from build123d import *

# Parameters (mm, degrees)
F0_R     = 11.125
F1_DEPTH = 7.5
F2_SIZE  = 1.524


with BuildPart() as f1:
    # F0 (on Top) → F1 (new body)
    with BuildSketch(Plane.XY):
        with BuildLine():
            ThreePointArc((13.1013648304, -5.7309894069), (13.9971339401, -2.9274974745), (14.3, 0))
            ThreePointArc((14.3, 0), (10.6581248351, 9.5338541524), (1.5875, 14.2116094708))
            Line((1.5875, 14.2116094708), (1.5875, 12.7125))
            Line((1.5875, 12.7125), (-1.5875, 12.7125))
            Line((-1.5875, 12.7125), (-1.5875, 14.2116094708))
            ThreePointArc((-1.5875, 14.2116094708), (-12.3841632741, 7.15), (-13.1013648304, -5.7309894069))
            Line((-13.1013648304, -5.7309894069), (-11.8030979456, -4.9814346715))
            Line((-11.8030979456, -4.9814346715), (-10.2155979456, -7.7310653285))
            Line((-10.2155979456, -7.7310653285), (-11.5138648304, -8.4806200639))
            ThreePointArc((-11.5138648304, -8.4806200639), (0, -14.3), (11.5138648304, -8.4806200639))
            Line((11.5138648304, -8.4806200639), (10.2155979456, -7.7310653285))
            Line((10.2155979456, -7.7310653285), (11.8030979456, -4.9814346715))
            Line((11.8030979456, -4.9814346715), (13.1013648304, -5.7309894069))
        make_face()
        Circle(F0_R, mode=Mode.SUBTRACT)
        with BuildLine():
            Line((1.5875, 12.7125), (1.5875, 14.2116094708))
            ThreePointArc((1.5875, 14.2116094708), (0, 14.3), (-1.5875, 14.2116094708))
            Line((-1.5875, 14.2116094708), (-1.5875, 12.7125))
            Line((-1.5875, 12.7125), (1.5875, 12.7125))
        make_face()
        with BuildLine():
            ThreePointArc((-1.5875, 14.2116094708), (0, 14.3), (1.5875, 14.2116094708))
            Line((1.5875, 14.2116094708), (1.5875, 17.5383905292))
            ThreePointArc((1.5875, 17.5383905292), (0, 17.45), (-1.5875, 17.5383905292))
            Line((-1.5875, 17.5383905292), (-1.5875, 14.2116094708))
        make_face()
        with BuildLine():
            Line((15.9824417398, -7.3943799361), (13.1013648304, -5.7309894069))
            ThreePointArc((13.1013648304, -5.7309894069), (12.3841632741, -7.15), (11.5138648304, -8.4806200639))
            Line((11.5138648304, -8.4806200639), (14.3949417398, -10.1440105931))
            ThreePointArc((14.3949417398, -10.1440105931), (15.112143296, -8.725), (15.9824417398, -7.3943799361))
        make_face()
        with BuildLine():
            ThreePointArc((11.5138648304, -8.4806200639), (12.3841632741, -7.15), (13.1013648304, -5.7309894069))
            Line((13.1013648304, -5.7309894069), (11.8030979456, -4.9814346715))
            Line((11.8030979456, -4.9814346715), (10.2155979456, -7.7310653285))
            Line((10.2155979456, -7.7310653285), (11.5138648304, -8.4806200639))
        make_face()
        with BuildLine():
            Line((1.5875, 19.0375), (1.5875, 17.5383905292))
            ThreePointArc((1.5875, 17.5383905292), (10.6581248351, 22.2161458476), (14.3, 31.75))
            ThreePointArc((14.3, 31.75), (-9.5338541524, 42.4081248351), (-1.5875, 17.5383905292))
            Line((-1.5875, 17.5383905292), (-1.5875, 19.0375))
            Line((-1.5875, 19.0375), (1.5875, 19.0375))
        make_face()
        with Locations((0, 31.75)):
            Circle(F0_R, mode=Mode.SUBTRACT)
        with BuildLine():
            ThreePointArc((-1.5875, 17.5383905292), (0, 17.45), (1.5875, 17.5383905292))
            Line((1.5875, 17.5383905292), (1.5875, 19.0375))
            Line((1.5875, 19.0375), (-1.5875, 19.0375))
            Line((-1.5875, 19.0375), (-1.5875, 17.5383905292))
        make_face()
        with BuildLine():
            Line((17.2807086245, -8.1439346715), (15.9824417398, -7.3943799361))
            ThreePointArc((15.9824417398, -7.3943799361), (15.112143296, -8.725), (14.3949417398, -10.1440105931))
            Line((14.3949417398, -10.1440105931), (15.6932086245, -10.8935653285))
            Line((15.6932086245, -10.8935653285), (17.2807086245, -8.1439346715))
        make_face()
        with BuildLine():
            ThreePointArc((41.7963065702, -15.875), (31.9595863578, -2.2893776905), (15.9824417398, -7.3943799361))
            Line((15.9824417398, -7.3943799361), (17.2807086245, -8.1439346715))
            Line((17.2807086245, -8.1439346715), (15.6932086245, -10.8935653285))
            Line((15.6932086245, -10.8935653285), (14.3949417398, -10.1440105931))
            ThreePointArc((14.3949417398, -10.1440105931), (24.5688090957, -29.8721339401), (41.7963065702, -15.875))
        make_face()
        with Locations((27.4963065702, -15.875)):
            Circle(F0_R, mode=Mode.SUBTRACT)
        with BuildLine():
            Line((-11.8030979456, -4.9814346715), (-13.1013648304, -5.7309894069))
            ThreePointArc((-13.1013648304, -5.7309894069), (-12.3841632741, -7.15), (-11.5138648304, -8.4806200639))
            Line((-11.5138648304, -8.4806200639), (-10.2155979456, -7.7310653285))
            Line((-10.2155979456, -7.7310653285), (-11.8030979456, -4.9814346715))
        make_face()
        with BuildLine():
            ThreePointArc((-11.5138648304, -8.4806200639), (-12.3841632741, -7.15), (-13.1013648304, -5.7309894069))
            Line((-13.1013648304, -5.7309894069), (-15.9824417398, -7.3943799361))
            ThreePointArc((-15.9824417398, -7.3943799361), (-15.112143296, -8.725), (-14.3949417398, -10.1440105931))
            Line((-14.3949417398, -10.1440105931), (-11.5138648304, -8.4806200639))
        make_face()
        with BuildLine():
            Line((-17.2807086245, -8.1439346715), (-15.9824417398, -7.3943799361))
            ThreePointArc((-15.9824417398, -7.3943799361), (-41.0819288797, -20.3382797877), (-13.1963065702, -15.875))
            ThreePointArc((-13.1963065702, -15.875), (-13.4991726301, -12.9475025255), (-14.3949417398, -10.1440105931))
            Line((-14.3949417398, -10.1440105931), (-15.6932086245, -10.8935653285))
            Line((-15.6932086245, -10.8935653285), (-17.2807086245, -8.1439346715))
        make_face()
        with Locations((-27.4963065702, -15.875)):
            Circle(F0_R, mode=Mode.SUBTRACT)
        with BuildLine():
            ThreePointArc((-14.3949417398, -10.1440105931), (-15.112143296, -8.725), (-15.9824417398, -7.3943799361))
            Line((-15.9824417398, -7.3943799361), (-17.2807086245, -8.1439346715))
            Line((-17.2807086245, -8.1439346715), (-15.6932086245, -10.8935653285))
            Line((-15.6932086245, -10.8935653285), (-14.3949417398, -10.1440105931))
        make_face()
    extrude(amount=F1_DEPTH)

    # F2
    f2_edges = [f1.edges().sort_by_distance(p)[0] for p in [
        (12.384163, 7.15, 7.5),
        (1.5875, 15.875, 7.5),
        (0, 46.05, 7.5),
        (-1.5875, 15.875, 7.5),
        (-12.384163, 7.15, 7.5),
        (-14.541903, -6.562685, 7.5),
        (-39.88047, -23.025, 7.5),
        (-12.954403, -9.312315, 7.5),
        (0, -14.3, 7.5),
        (12.954403, -9.312315, 7.5),
        (39.88047, -23.025, 7.5),
        (14.541903, -6.562685, 7.5),
        (-11.125, 0, 7.5),
        (-11.125, 31.75, 7.5),
        (16.371307, -15.875, 7.5),
        (-38.621307, -15.875, 7.5),
        (12.384163, 7.15, 0),
        (1.5875, 15.875, 0),
        (0, 46.05, 0),
        (-1.5875, 15.875, 0),
        (-12.384163, 7.15, 0),
        (-14.541903, -6.562685, 0),
        (-39.88047, -23.025, 0),
        (-12.954403, -9.312315, 0),
        (0, -14.3, 0),
        (12.954403, -9.312315, 0),
        (39.88047, -23.025, 0),
        (14.541903, -6.562685, 0),
        (-11.125, 0, 0),
        (-11.125, 31.75, 0),
        (16.371307, -15.875, 0),
        (-38.621307, -15.875, 0),
    ]]
    chamfer(f2_edges, length=F2_SIZE)


solid = f1.part
Design review of the part built by this model. Coordinates are the model's own, in mm. A direction names the side the tool comes from. Round coordinates to 2 decimals unless told otherwise and drop trailing zeros. Use a Markdown table: item, result. Add a question column.
1. Clearance check with flat-ended pins moving along their axes: pin 1 (1.5 mm diameter, centred on x = 18.5, z = 6.5, fed in from -Y); pin 2 (3 mm diameter, centred on x = -16.5, z = 6, fed in from +Y); pin 3 (20 mm diameter, centred on x = 0, y = 0, fed in from +Z); pin 4 (2 mm diameter, centred on x = 16.5, z = 3, fed in from +Y). State where each tip first meets the part, or that it passes through.
2. We need section A-A (z = 2.5). Count the separate pieces of the cut face and the enclosed holes in it, then the cut area to 3 significant figures.
3. Mouldability with a two-part tool opening along Y and no side actions: class faces 1 (the face through (12.93, -9.3, 3.72)), 2 (the face through (-0.19, -13.018, 0.243)) as +Y half, -Y half, draft (parallel to the pull), parting line (faces both ways), or undercut.
4. For faces 3 (the face through (14.562, -6.574, 3.719)), 4 (the face through (-13.378, -8.665, 0.751)), 5 (the face through (14.19, -7.25, 6.75)), 6 (the face through (1.588, 16, 4)), 7 (the face through (-1.588, 16, 4)), list the 3-axis set-ups (+Z, -Z, +X, -X, +Y, -Y) from which the entire face can be reached by the end or side of a thin tool; tool diameter is ignored.
5. Wall thickness on probe 1 along Y at (x, z) = (0, 2.8) (3 decimals); probe 2 along Y at (x, z) = (28, 2.25); probe 3 along X at (y, z) = (-15, 4.75): over which ranges is each line inside the solid? List them lowest first.
Output:
| question | item | result |
|---|---|---|
| 1 | pin 1 | stops at y = -27.4 |
| 1 | pin 2 | stops at y = -5.18 |
| 1 | pin 3 | passes through |
| 1 | pin 4 | stops at y = -5.65 |
| 2 | separate pieces | 1 |
| 2 | enclosed holes | 4 |
| 2 | area | 1,040 mm2 |
| 3 | face 1 | undercut |
| 3 | face 2 | -Y half |
| 4 | face 3 | +Z, -Z |
| 4 | face 4 | -Z |
| 4 | face 5 | +Z |
| 4 | face 6 | +Z, -Z, +X |
| 4 | face 7 | +Z, -Z, -X |
| 5 | probe 1 | y = -14.3 to -11.125, 11.125 to 20.625, 42.875 to 46.05 |
| 5 | probe 2 | y = -30.17 to -26.99, -4.76 to -1.58 |
| 5 | probe 3 | x = -41.77 to -38.59, -16.41 to -13.22, 13.22 to 16.41, 38.59 to 41.77 |
